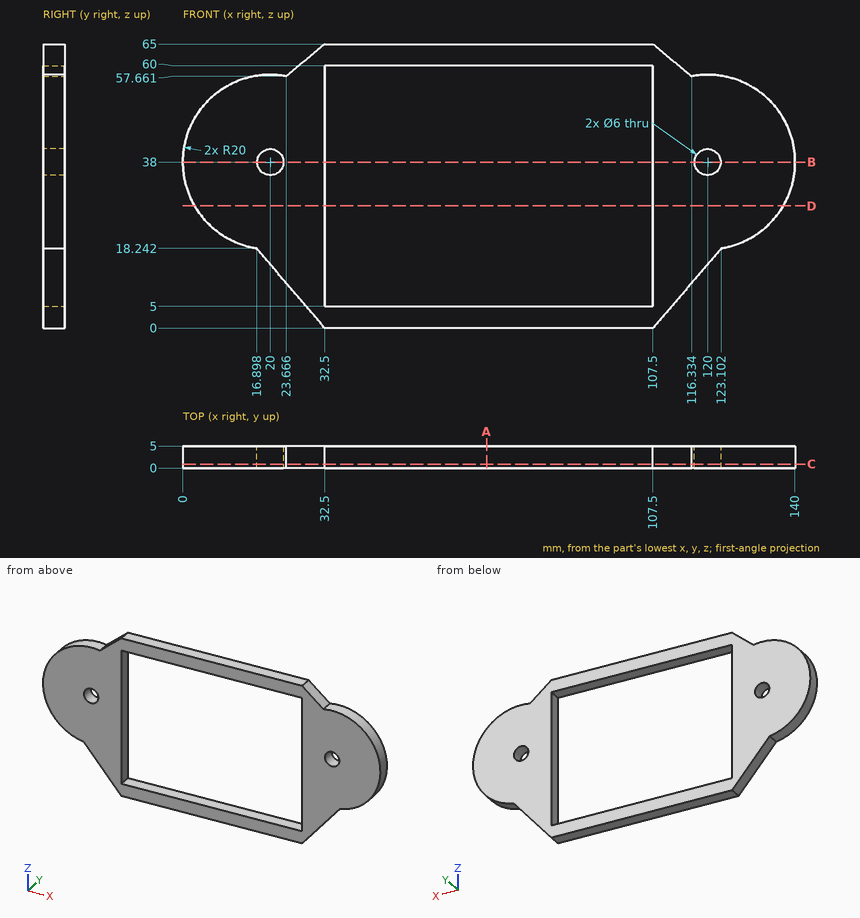
Source: three-view drawing plus pictorial views. Frame: mm from the lowest corner of the part. Give positions to 0.01 mm unless a question says otherwise; leave off trailing zeros. Order: outer loops, then holes, each group sorted by start corner. A loop starts at its lowest first (then second) coordinate and runs counter-clockwise, first axis right, second up. Notation, with made-up numbers: M 6.25,12.5 L 36.25,12.5 A30 cw 36.25,35.5 Z; hole C 51,1 d1. An arc over 180 degrees is marked long. Return JSON: item names as keys, results as strings.
1) Line query: L1, parallel to Z at x = 50, y = 1.55; L2, parallel to X at y = 4.8, z = 22.5; L3, parallel to X at y = 3.25, z = 55 (1 decimal). Output: solid intervals per line, ascending. Write a range as [from, to].
Taken from the geometry:
{"L1": "z = [0, 5], [60, 65]", "L2": "x = [7.36, 32.5], [107.5, 132.64]", "L3": "x = [9.5, 32.5], [107.5, 130.5]"}
2) Section query B-B on z = 38. Output: boundary loops of the cut face in (x, y), and give its area (3 significant figures).
Taken from the geometry:
{"outline": "M 0,0 L 17,0 L 17,5 L 0,5 Z; M 23,0 L 32.5,0 L 32.5,5 L 23,5 Z; M 107.5,0 L 117,0 L 117,5 L 107.5,5 Z; M 123,0 L 140,0 L 140,5 L 123,5 Z", "area": "265 mm2"}
3) Contact query for flat-ended pins moving along their axis: pin 1 (5.5 mm diameter, centred on x = 20, z = 38, fed in from -Y); pin 2 (1.5 mm diameter, centred on y = 2.5, z = 40.5, fed in from -X). Output: stop coordinate, or through.
Taken from the geometry:
{"pin 1": "passes through", "pin 2": "stops at x = 0.08"}
4) Section query D-D on z = 28. Output: boundary loops of the cut face in (x, y), and give its area (3 significant figures).
Taken from the geometry:
{"outline": "M 2.68,0 L 32.5,0 L 32.5,5 L 2.68,5 Z; M 107.5,0 L 137.32,0 L 137.32,5 L 107.5,5 Z", "area": "298 mm2"}
5) Section query C-C on y = 0.9. Output: boundary loops of the cut face in (x, z).
Taken from the geometry:
{"outline": "M 16.9,18.24 L 32.5,0 L 107.5,0 L 123.1,18.24 A20 ccw long 116.33,57.66 L 107.5,65 L 32.5,65 L 23.67,57.66 A20 ccw long Z; hole C 20,38 d6; hole M 32.5,5 L 107.5,5 L 107.5,60 L 32.5,60 Z; hole C 120,38 d6"}
6) Section query A-A on x = 69.5. Output: boundary loops of the cut face in (y, z).
Taken from the geometry:
{"outline": "M 0,0 L 5,0 L 5,5 L 0,5 Z; M 0,60 L 5,60 L 5,65 L 0,65 Z"}
